Input: dimensioned drawing with shaded views. Units: mm. Origin: part minimum x, y, z. Give positions to 0.01 mm unless a question says otherwise; leave off trailing zeros. Write each loop counter-clockwise with the first axis right and the second up, starting at its lowest first coordinate (ties: lowest second). Pieces come first, ordered by that corner, then holes. Notation, with made-up numbers: M 57,14 L 112,14 A26 cw 112,29 Z; hole C 11,-4.5 d2. An arc over 180 degrees is marked long. Answer as a JSON object with one key per item and string values.
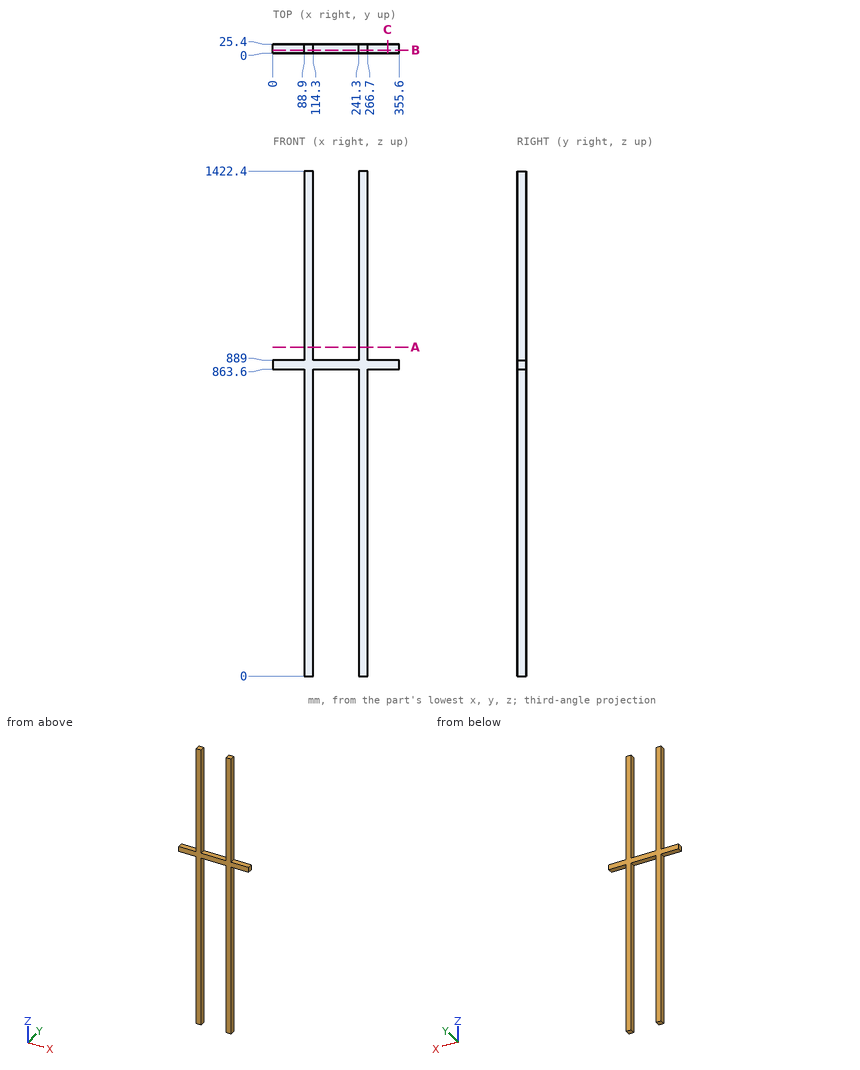
1) Cut plane B-B on y = 8.25. Return loops of the section in (x, z), and give its area (3 significant figures).
Geometry check:
{"outline": "M 0,863.6 L 88.9,863.6 L 88.9,0 L 114.3,0 L 114.3,863.6 L 241.3,863.6 L 241.3,0 L 266.7,0 L 266.7,863.6 L 355.6,863.6 L 355.6,889 L 266.7,889 L 266.7,1422.4 L 241.3,1422.4 L 241.3,889 L 114.3,889 L 114.3,1422.4 L 88.9,1422.4 L 88.9,889 L 0,889 Z", "area": "80,000 mm2"}
2) Contact query for flat-ended pins moving along their axis: P1, Ø12.5, axis at x = 34, y = 13, coming from the +Z side; P2, Ø10, axis at x = 71, y = 19, coming from the -Z side; P3, Ø2, axis at y = 6.5, z = 384, coming from the +X side. Output: stop coordinate, or through.
Geometry check:
{"P1": "stops at z = 889", "P2": "stops at z = 863.6", "P3": "stops at x = 266.7"}
3) Line query: line 1 (X direction, y = 18.75, z = 484); line 2 (Z direction, x = 189, y = 10.5). Output: solid intervals per line, ascending. Write a range as from..to.
Geometry check:
{"line 1": "x = 88.9..114.3, 241.3..266.7", "line 2": "z = 863.6..889"}
4) Cut plane C-C on x = 323. Return loops of the section in (y, z).
Geometry check:
{"outline": "M 0,863.6 L 25.4,863.6 L 25.4,889 L 0,889 Z"}
5) Cut plane A-A on z = 926. Return loops of the section in (x, y).
Geometry check:
{"outline": "M 88.9,0 L 114.3,0 L 114.3,25.4 L 88.9,25.4 Z; M 241.3,0 L 266.7,0 L 266.7,25.4 L 241.3,25.4 Z"}
